Can you work these out from the model? Positions are in its coordinate system, mm. Face numbers are marked on the shaded views. A direction names the side the tool comes from. Give positions to 0.01 mm unless a question says otherwise; leave off trailing zeros. Loops run counter-clockwise (first coordinate to the right, second up) from the corner with the lowest first, then second, coordinate; pieces in that order, holes last. Notation, with made-up numbers: (17.25, 71) -> (45.25, 71) arc R28 cw to (45.25, 99) -> close; hole circle Ø6 at (15.5, 56). An arc over 180 degrees is marked (long way). Use CSV: the item, a comma, the result in double quotes.
from build123d import *

# Parameters (mm, degrees)
F0_W     = 50.8
F0_H     = 101.6
F1_DEPTH = 12.7
F2_W     = 19.05
F2_H     = 50.8
F3_DEPTH = 44.45
F5_DEPTH = 9.652
F7_D     = 22.352


with BuildPart() as f1:
    # F0 (on Top) → F1 (new body)
    with BuildSketch(Plane.XY):
        with Locations((0.128248, -50.8)):
            Rectangle(F0_W, F0_H)
    extrude(amount=F1_DEPTH)

    # F2 (on face) → F3 (join)
    with BuildSketch(Plane.XY.offset(12.7)):
        with Locations((-15.746752, -25.4)):
            Rectangle(F2_W, F2_H)
    extrude(amount=F3_DEPTH)

    # F4 (on face) → F5 (join)
    with BuildSketch(Plane(origin=(0, 0, 0), x_dir=(-1, 0, 0), z_dir=(0, 1, 0))):
        Polygon((6.221752, 12.7), (6.221752, 57.15), (-25.528248, 12.7), align=None)
    extrude(amount=-F5_DEPTH)

    # F7 (through all)
    with Locations(Plane.YZ.offset(-6.221752)):
        with Locations((-35.627518, 36.184873)):
            Hole(F7_D / 2)


solid = f1.part
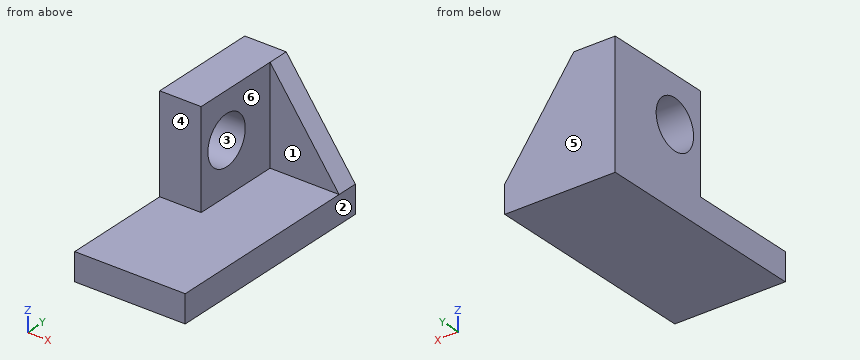
(1) If we section it at C-C, the plane x = -10.5: Write out the boundary of the cut face in (y, z).
Answer sheet:
outline,"(-101.6, 0) -> (0, 0) -> (0, 57.15) -> (-50.8, 57.15) -> (-50.8, 12.7) -> (-101.6, 12.7) -> close; hole circle Ø22.35 at (-35.63, 36.18)"
(2) If we section it at B-B, the plane y = -32: Write out the boundary of the cut face in (x, z).
Answer sheet:
outline,"(-25.27, 0) -> (25.53, 0) -> (25.53, 12.7) -> (-6.22, 12.7) -> (-6.22, 25.61) -> (-25.27, 25.61) -> close; (-25.27, 46.76) -> (-6.22, 46.76) -> (-6.22, 57.15) -> (-25.27, 57.15) -> close"
(3) Which directions (+Z, -Z, +X, -X, +Y, -Y) give clear straight access to the entire face, cutting with the end or side of a thin tool? Please do the marked faces 4, 5 and 6.
Answer sheet:
face 4,"+Z, +X, -X, -Y"
face 5,"+Z, -Z, +X, -X, +Y"
face 6,"+Z, +X, -Y"
(4) If I drill on L1, parallel to Z at x = 0, y = -92; L2, parallel to Y at x = 7, z = 13.5; L3, parallel to Y at x = -21.5, z = 20, over which ranges is the centre line in solid material (lowest first)? Write a range as from..to.
Answer sheet:
L1,"z = 0..12.7"
L2,"y = -9.65..0"
L3,"y = -50.8..0"
(5) If we section it at D-D, the plane y = -21.5: Write out the boundary of the cut face in (x, z), then the cut area to 3 significant figures.
Answer sheet:
outline,"(-25.27, 0) -> (25.53, 0) -> (25.53, 12.7) -> (-6.22, 12.7) -> (-6.22, 57.15) -> (-25.27, 57.15) -> close"
area,"1,490 mm2"
(6) We'd pull the mould along Y, two halves only. Please class the marked faces 1, 2 and 3: released by +Y, released by -Y, zero draft, split by the parting line, or undercut.
Answer sheet:
face 1,"released by -Y"
face 2,"zero draft"
face 3,"undercut"
(7) Will these pins go through, and if not, where does the flat tip stop? pin 1 Ø5 at (x, y) = (3, -17.5) entering from +Z; pin 2 Ø15 at (x, z) = (-18.5, 27.5) entering from -Y.
Answer sheet:
pin 1,"stops at z = 12.7"
pin 2,"stops at y = -50.8"
(8) If we section it at A-A, the plane z = 28: Write out the boundary of the cut face in (x, y), then the cut area to 3 significant figures.
Answer sheet:
outline,"(-25.27, -50.8) -> (-6.22, -50.8) -> (-6.22, -43.24) -> (-25.27, -43.24) -> close; (-25.27, -28.02) -> (-6.22, -28.02) -> (-6.22, -9.65) -> (14.6, -9.65) -> (14.6, 0) -> (-25.27, 0) -> close"
area,"879 mm2"
